Input: part model. Units: mm. Frame: model coordinates. Face numbers are marked on the shaded views. A direction names the side the tool comes from. Give positions to 0.01 mm unless a question says otherwise; leave off trailing zeros. Loops run counter-clockwise (first coordinate to the right, second up) from the corner with the lowest first, then second, coordinate; pieces in that order, holes last. Notation, with made-up numbers: (65, -11) - (98, -11) arc R20 ccw to (98, -6) - close; hole circle Ø8 at (79, -15). An arc over 180 degrees is marked (long way). Answer as a JSON object with one key per item and string values.
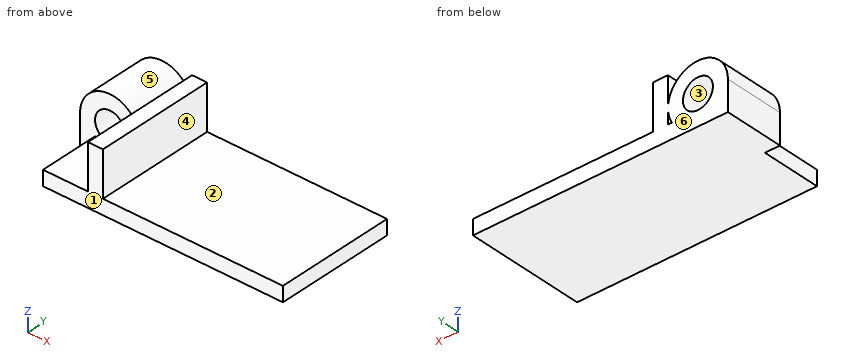
Autodesk Inventor part; units mm, degrees
ref_plane "YZ Plane" through (0, 0, 0) normal (1, 0, 0) x (0, 1, 0)
ref_plane "XZ Plane" through (0, 0, 0) normal (0, 1, 0) x (-1, 0, 0)
ref_plane "XY Plane" through (0, 0, 0) normal (0, 0, 1) x (1, 0, 0)
sketch "Sketch1" plane through (0, 0, 0) normal (0, 0, 1) x (1, 0, 0)
  line L0 (-11.9535, 4.9767) -> (38.8465, 4.9767)
  line L1 (38.8465, 4.9767) -> (38.8465, -20.4233)
  line L2 (38.8465, -20.4233) -> (-11.9535, -20.4233)
  line L3 (-11.9535, -20.4233) -> (-11.9535, 4.9767)
  point P0 (0, 0)
  dimension "d0" = 50.8
  dimension "d1" = 25.4
extrude "Extrusion1" add sketch "Sketch1" along normal blind 3.175
sketch "Sketch2" plane through (-11.9535, 4.9767, 0) normal (0, 1, 0) x (1, 0, 0)
  line L0 (0, -3.175) -> (50.8, -3.175)
  line L1 (0, -3.175) -> (3.175, -3.175)
  line L2 (3.175, -3.175) -> (3.175, -6.35)
  circle A0 centre (3.175, -6.35) radius 3.175
  circle A1 centre (3.175, -6.35) radius 4.4901
  point P0 (11.9535, 0)
  dimension "d4" = 3.175
  dimension "d5" = 3.175
extrude "Extrusion2" add sketch "Sketch2" against normal blind 12.7
sketch "Sketch3" plane through (-11.9535, 4.9767, 0) normal (0, 1, 0) x (1, 0, 0)
  line L0 (6.35, -3.175) -> (50.8, -3.175)
  arc A0 (0, -3.175) -> (6.35, -3.175) centre (3.175, -6.35) ccw
  line L1 (7.6651, -6.35) -> (7.6651, -3.175)
  point P0 (11.9535, 0)
extrude "Extrusion3" add sketch "Sketch3" against normal blind 12.7
sketch "Sketch4" plane through (-11.9535, 4.9767, 0) normal (0, 1, 0) x (1, 0, 0)
  line L0 (7.6651, -3.175) -> (50.8, -3.175)
  line L1 (50.8, 0) -> (50.8, -3.175)
  line L2 (0, 0) -> (50.8, 0)
  line L3 (0, 0) -> (0, -3.175)
  arc A0 (0, -3.175) -> (7.6651, -6.35) centre (3.175, -6.35) ccw
  line L4 (7.6651, -6.35) -> (7.6651, -3.175)
  line L5 (7.6651, -3.175) -> (7.6651, -12.2458)
  line L6 (3.175, -10.8401) -> (7.6651, -10.8401)
  point P0 (11.9535, 0)
extrude "Extrusion4" add sketch "Sketch4" against normal blind 12.7 contours L5 L6 A0
sketch "Sketch5" plane through (-11.9535, 4.9767, 0) normal (0, 1, 0) x (1, 0, 0)
  arc A0 (0, -3.175) -> (3.175, -10.8401) centre (3.175, -6.35) ccw
  line L0 (3.175, -10.8401) -> (7.6651, -10.8401)
  line L1 (7.6651, -10.8401) -> (7.6651, -3.175)
  circle A1 centre (3.175, -6.35) radius 3.175
  line L2 (7.6651, -3.175) -> (0, -3.175)
  point P0 (11.9535, 0)
extrude "Extrusion5" cut sketch "Sketch5" against normal blind 25.4
sketch "Sketch6" plane through (-11.9535, 4.9767, 0) normal (0, 1, 0) x (1, 0, 0)
  line L0 (0, -3.175) -> (50.8, -3.175)
  line L1 (0, 0) -> (50.8, 0)
  line L2 (0, -3.175) -> (3.175, -3.175)
  line L3 (3.175, -3.175) -> (3.175, -6.35)
  circle A0 centre (3.175, -6.35) radius 3.175
  circle A1 centre (3.175, -6.35) radius 6.35
  point P0 (11.9535, 0)
  dimension "d14" = 3.175
  dimension "d15" = 3.175
extrude "Extrusion6" add sketch "Sketch6" against normal blind 12.7
sketch "Sketch7" plane through (-11.9535, 4.9767, 0) normal (0, 1, 0) x (1, 0, 0)
  line L0 (0, 0) -> (0, -0.8507)
  arc A0 (0, -0.8507) -> (8.6743, -3.175) centre (3.175, -6.35) ccw
  line L1 (-3.175, -6.35) -> (-3.175, 0)
  line L2 (0, 0) -> (-3.175, 0)
  point P0 (11.9535, 0)
extrude "Extrusion7" add sketch "Sketch7" against normal blind 12.7
sketch "Sketch8" plane through (-11.9535, -20.4233, 0) normal (0, -1, 0) x (1, 0, 0)
  line L0 (50.8, 3.175) -> (0, 3.175)
  line L1 (0, 3.175) -> (6.35, 3.175)
  line L2 (6.35, 3.175) -> (9.525, 3.175)
  line L3 (9.525, 3.175) -> (9.525, 12.7)
  line L4 (9.525, 12.7) -> (12.7, 12.7)
  line L5 (12.7, 12.7) -> (12.7, 3.175)
  line L6 (12.7, 3.175) -> (9.525, 3.175)
  line L7 (9.525, 3.175) -> (9.525, 12.7)
  point P0 (11.9535, 0)
  dimension "d20" = 6.35
  dimension "d21" = 3.175
  dimension "d22" = 9.525
  dimension "d23" = 3.175
extrude "Extrusion8" add sketch "Sketch8" against normal blind 25.4
properties part number "hingely"
Item 1: Contact query for flat-ended pins moving along their axis: P1, Ø12.5, axis at x = 12, y = -5, coming from the +Z side (3 decimals); P2, Ø1, axis at x = 2.5, z = 7, coming from the +Y side; P3, Ø1.6, axis at y = -11, z = 1.5, coming from the -X side; P4, Ø4, axis at x = -9, z = 8.5, coming from the -Y side. Output: stop coordinate, or through.
Geometry check:
{"P1": "stops at z = 3.175", "P2": "passes through", "P3": "stops at x = -11.95", "P4": "stops at y = -7.72"}
Item 2: Access query for the marked faces 1 and 2. Directions: +Z, -Z, +X, -X, +Y, -Y. A direction counts if a zero-diameter tool reaches every point of the face in a straight line with its end or side. Return the directions, or none.
Geometry check:
{"face 1": "+Z, -Z, +X, -X, -Y", "face 2": "+Z, +X, +Y, -Y"}
Item 3: Cut plane C-C (x = -4). Return loops of the section in (y, z) (3 decimals), then the cut area to 3 significant figures.
Geometry check:
{"outline": "(-20.423, 0) - (4.977, 0) - (4.977, 10.532) - (-7.723, 10.532) - (-7.723, 3.175) - (-20.423, 3.175) - close", "area": "174 mm2"}
Item 4: Mould query, pull axis X, two halves, no side actions, for the marked faces 3, 4, 5 and 6. Classes: released by +X, released by -X, zero draft, split by the parting line, or undercut.
Geometry check:
{"face 3": "undercut", "face 4": "released by +X", "face 5": "undercut", "face 6": "zero draft"}
Item 5: Material intervals for line 1 (Z direction, x = 29, y = -18.75) (3 decimals); line 2 (X direction, y = -16, z = 12.25); line 3 (X direction, y = -12, z = 2.5), sorted ascending. Write a range as [from, to].
Geometry check:
{"line 1": "z = [0, 3.175]", "line 2": "x = [-2.43, 0.75]", "line 3": "x = [-11.95, 38.85]"}
Item 6: Cut plane D-D (x = 16). Return loops of the section in (y, z) (3 decimals).
Geometry check:
{"outline": "(-20.423, 0) - (4.977, 0) - (4.977, 3.175) - (-20.423, 3.175) - close"}
Item 7: Cut plane A-A (y = -16.25). Return loops of the section in (x, z) (1 decimal).
Geometry check:
{"outline": "(-12, 0) - (38.8, 0) - (38.8, 3.2) - (0.7, 3.2) - (0.7, 12.7) - (-2.4, 12.7) - (-2.4, 3.2) - (-12, 3.2) - close"}
Item 8: Cut plane B-B (z = 4). Return loops of the section in (x, y), then the cut area to 3 significant figures.
Geometry check:
{"outline": "(-15.13, -7.72) - (-10.91, -7.72) - (-10.91, 4.98) - (-15.13, 4.98) - close; (-6.64, -7.72) - (-2.88, -7.72) - (-2.88, 4.98) - (-6.64, 4.98) - close; (-2.43, -20.42) - (0.75, -20.42) - (0.75, 4.98) - (-2.43, 4.98) - close", "area": "182 mm2"}
